Model file for the job. Use its own axes, mm. Face numbers are marked on the shaded views. A direction names the side the tool comes from. Round coordinates to 2 decimals unless told otherwise and drop trailing zeros. Write each loop counter-clockwise with the first axis right and the second up, starting at its lowest first coordinate (ties: lowest second). Pieces come first, ordered by that corner, then holes. Notation, with made-up numbers: (62.25, 55.5) - (95.25, 55.5) arc R24 ccw to (95.25, 83.5) - close; hole circle Ø2 at (4, 82.5). An arc over 180 degrees is marked (long way). One line per item, written item: value.
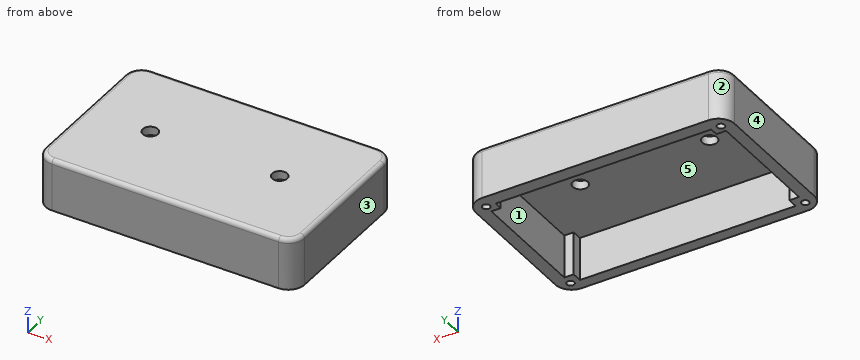
from build123d import *

# Parameters (mm, degrees)
F0_W         = 120
F0_H         = 75
F1_DEPTH     = 4
F2_W         = 120
F2_H         = 75
F3_DEPTH     = 20
F4_R         = 2
F5_T1_DEPTH  = 42.75
F5_T4_ANGLE  = 90
F5_T6_ANGLE  = 90
F5_T8_ANGLE  = 90
F5_T10_ANGLE = 90
F6_R         = 3.5
F7_DEPTH     = 25
F8_R         = 1.7577503979
F8_R_2       = 1.75
F9_DEPTH     = 10


# Not quite as in the source:
# - a fillet or chamfer that OpenCascade refuses, or shapes differently, is made with other operations: its cross-section is extruded or revolved along the edge and cut away or added


with BuildPart() as f1:
    # F0 (on Top) → F1 (new body)
    with BuildSketch(Plane.XY):
        Rectangle(F0_W, F0_H)
    extrude(amount=F1_DEPTH)

    # F2 (on face) → F3 (join)
    with BuildSketch(Plane(origin=(0, 0, 0), x_dir=(1, 0, 0), z_dir=(0, 0, -1))):
        Rectangle(F2_W, F2_H)
        Polygon((54.339364171, -27.5), (50, -27.5), (50, -31.3459709287), (-50, -31.3459709287), (-50, -27.5), (-54.5065030456, -27.5), (-54.5065030456, 27.5), (-50, 27.5), (-50, 32.2239883244), (50, 32.2239883244), (50, 27.5), (54.339364171, 27.5), align=None, mode=Mode.SUBTRACT)
    extrude(amount=F3_DEPTH)

    # F4
    f4_edges = [f1.edges().sort_by_distance(p)[0] for p in [
        (60, 0, 4),
        (0, -37.5, 4),
        (-60, 0, 4),
        (0, 37.5, 4),
    ]]
    fillet(f4_edges, radius=F4_R)

    # F5: fillet of radius 7.5 on 4 edges, made by hand

    # F5_s2 → F5_t1 (cut)
    with BuildSketch(Plane.XY.offset(-38.75)):
        with BuildLine():
            ThreePointArc((60, -30), (57.8033008589, -35.3033008589), (52.5, -37.5))
            Line((52.5, -37.5), (60, -37.5))
            Line((60, -37.5), (60, -30))
        make_face()
        with BuildLine():
            ThreePointArc((60, 30), (57.8033008589, 35.3033008589), (52.5, 37.5))
            Line((52.5, 37.5), (60, 37.5))
            Line((60, 37.5), (60, 30))
        make_face()
        with BuildLine():
            ThreePointArc((-52.5, -37.5), (-57.8033008589, -35.3033008589), (-60, -30))
            Line((-60, -30), (-60, -37.5))
            Line((-60, -37.5), (-52.5, -37.5))
        make_face()
        with BuildLine():
            ThreePointArc((-52.5, 37.5), (-57.8033008589, 35.3033008589), (-60, 30))
            Line((-60, 30), (-60, 37.5))
            Line((-60, 37.5), (-52.5, 37.5))
        make_face()
    extrude(amount=F5_T1_DEPTH, mode=Mode.SUBTRACT)

    # F5_s3 → F5_t4 (revolve, cut)
    with BuildSketch(Plane.YZ.offset(-52.5)):
        with BuildLine():
            ThreePointArc((35.5, 4), (36.9142135624, 3.4142135624), (37.5, 2))
            Line((37.5, 2), (37.5, 4))
            Line((37.5, 4), (35.5, 4))
        make_face()
    revolve(axis=Axis((-52.5, 30, 4), (0, 0, 1)), revolution_arc=F5_T4_ANGLE, mode=Mode.SUBTRACT)

    # F5_s5 → F5_t6 (revolve, cut)
    with BuildSketch(Plane.XZ.offset(30)):
        with BuildLine():
            ThreePointArc((-58, 4), (-59.4142135624, 3.4142135624), (-60, 2))
            Line((-60, 2), (-60, 4))
            Line((-60, 4), (-58, 4))
        make_face()
    revolve(axis=Axis((-52.5, -30, 4), (0, 0, 1)), revolution_arc=F5_T6_ANGLE, mode=Mode.SUBTRACT)

    # F5_s7 → F5_t8 (revolve, cut)
    with BuildSketch(Plane.XZ.offset(-30)):
        with BuildLine():
            ThreePointArc((58, 4), (59.4142135624, 3.4142135624), (60, 2))
            Line((60, 2), (60, 4))
            Line((60, 4), (58, 4))
        make_face()
    revolve(axis=Axis((52.5, 30, 4), (0, 0, 1)), revolution_arc=F5_T8_ANGLE, mode=Mode.SUBTRACT)

    # F5_s9 → F5_t10 (revolve, cut)
    with BuildSketch(Plane.YZ.offset(52.5)):
        with BuildLine():
            ThreePointArc((-35.5, 4), (-36.9142135624, 3.4142135624), (-37.5, 2))
            Line((-37.5, 2), (-37.5, 4))
            Line((-37.5, 4), (-35.5, 4))
        make_face()
    revolve(axis=Axis((52.5, -30, 4), (0, 0, 1)), revolution_arc=F5_T10_ANGLE, mode=Mode.SUBTRACT)

    # F6 (on face) → F7 (cut)
    with BuildSketch(Plane.XY.offset(4)):
        with Locations((-30, 0)):
            Circle(F6_R)
        with Locations((30, 0)):
            Circle(F6_R)
    extrude(amount=-F7_DEPTH, mode=Mode.SUBTRACT)

    # F8 (on face) → F9 (cut)
    with BuildSketch(Plane(origin=(0, 0, -20), x_dir=(1, 0, 0), z_dir=(0, 0, -1))):
        with Locations((-54.5065030456, 32.2239883244)):
            Circle(F8_R)
        with Locations((54.339364171, 32.2239883244)):
            Circle(F8_R_2)
        with Locations((54.339364171, -31.3459709287)):
            Circle(F8_R_2)
        with Locations((-54.5065030456, -31.3459709287)):
            Circle(F8_R_2)
    extrude(amount=-F9_DEPTH, mode=Mode.SUBTRACT)


solid = f1.part
1. Drop flat-ended pins along their axis: pin 1 (9 mm diameter, centred on x = -30, y = 0, fed in from -Z); pin 2 (1 mm diameter, centred on x = 54.5, y = -32, fed in from -Z); pin 3 (4 mm diameter, centred on x = 30, y = 0, fed in from +Z). Give the stop position or say it passes through.
Report:
pin 1: z = 0
pin 2: z = -10
pin 3: through
2. Band-saw the part on A-A on y = 0. Write the cut outline in (x, z).
Report:
outline: (-60, -20) - (-54.51, -20) - (-54.51, 0) - (-33.5, 0) - (-33.5, 4) - (-58, 4) arc R2 ccw to (-60, 2) - close; (-26.5, 0) - (26.5, 0) - (26.5, 4) - (-26.5, 4) - close; (33.5, 0) - (54.34, 0) - (54.34, -20) - (60, -20) - (60, 2) arc R2 ccw to (58, 4) - (33.5, 4) - close
3. Band-saw the part on C-C on z = -7.75. Write the cut outline in (x, y), plus the area to 3 significant figures.
Report:
outline: (-60, -30) arc R7.5 ccw to (-52.5, -37.5) - (52.5, -37.5) arc R7.5 ccw to (60, -30) - (60, 30) arc R7.5 ccw to (52.5, 37.5) - (-52.5, 37.5) arc R7.5 ccw to (-60, 30) - close; hole (-54.51, -27.5) - (-50, -27.5) - (-50, -32.22) - (50, -32.22) - (50, -27.5) - (54.34, -27.5) - (54.34, 27.5) - (50, 27.5) - (50, 31.35) - (-50, 31.35) - (-50, 27.5) - (-54.51, 27.5) - close
area: 2,110 mm²
4. Wall check: probe 1 along X at (y, z) = (9, -12); probe 2 along Y at (x, z) = (30, 2.1); probe 3 along Y at (x, z) = (-38, -1.5). Give the ranges that are in metal, low to high. Write a range as [from, to].
Report:
probe 1: [-60, -54.51], [54.34, 60]
probe 2: [-37.5, -3.5], [3.5, 37.5]
probe 3: [-37.5, -32.22], [31.35, 37.5]
5. Band-saw the part on D-D on y = -18. Write the cut outline in (x, z), plus the area to 3 significant figures.
Report:
outline: (-60, -20) - (-54.51, -20) - (-54.51, 0) - (54.34, 0) - (54.34, -20) - (60, -20) - (60, 2) arc R2 ccw to (58, 4) - (-58, 4) arc R2 ccw to (-60, 2) - close
area: 701 mm²
6. Mould opens along X. For the marked faces 3, 4 and 5 say: released by +X, released by -X, zero draft, split by the parting line, or undercut.
Report:
face 3: released by +X
face 4: released by -X
face 5: undercut
7. Tool access for the marked faces 1 and 2: list every direction of +Z, -Z, +X, -X, +Y, -Y with a clear straight run to the whole face (end or side of a thin tool).
Report:
face 1: -Z
face 2: +Z, -Z, -X, +Y
8. Band-saw the part on B-B on x = 30. Write the cut outline in (y, z).
Report:
outline: (-37.5, -20) - (-32.22, -20) - (-32.22, 0) - (-3.5, 0) - (-3.5, 4) - (-35.5, 4) arc R2 ccw to (-37.5, 2) - close; (3.5, 0) - (31.35, 0) - (31.35, -20) - (37.5, -20) - (37.5, 2) arc R2 ccw to (35.5, 4) - (3.5, 4) - close
